Answer from the drawing. Dimensions are ordinates in mm from the lowest x, y and z of the part. Round coordinates to 2 decimals unless told otherwise and drop trailing zeros. Loops run counter-clockwise (first coordinate to the right, second up) from the corner with the lowest first, then second, coordinate; pieces in that order, holes last. Notation, with made-up numbers: (77.25, 1) - (121.25, 1) arc R27 ccw to (121.25, 17) - close; hole circle Ø11 at (-9, -6.75). An arc over 180 degrees is marked (long way). Return JSON: item names as keys, results as strings.
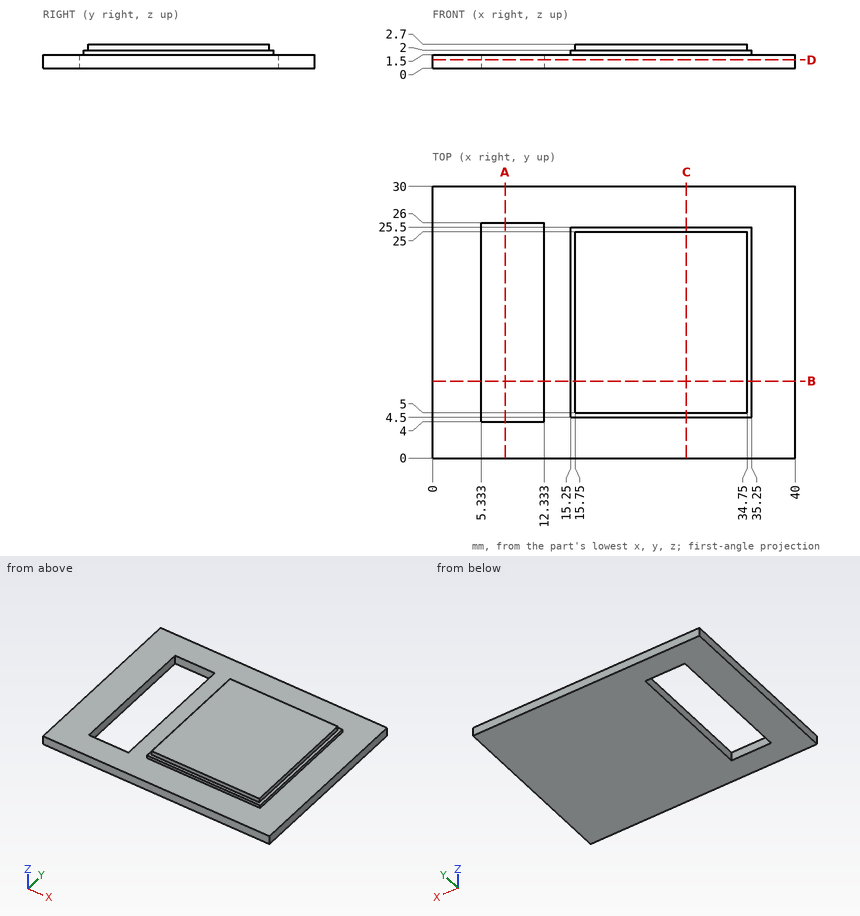
1) Flat-ended cylindrical pins translate along their axes: pin 1 (8 mm diameter, centred on x = 36, y = 14.5, fed in from +Z); pin 2 (8 mm diameter, centred on x = 6.5, y = 19, fed in from +Z); pin 3 (0.8 mm diameter, centred on x = 30, z = 2, fed in from -Y); pin 4 (0.6 mm diameter, centred on y = 11.5, z = 2, fed in from -X). Find the tip coordinate at first contact, or state that the pin passes through.
Verdict:
{"pin 1": "stops at z = 2.7", "pin 2": "stops at z = 1.5", "pin 3": "stops at y = 4.5", "pin 4": "stops at x = 15.25"}
2) Section C-C (x = 28) is taken. Give the vertices of the cut face in (y, z), and give its area (3 significant figures).
Verdict:
{"outline": "(0, 0) - (30, 0) - (30, 1.5) - (25.5, 1.5) - (25.5, 2) - (25, 2) - (25, 2.7) - (5, 2.7) - (5, 2) - (4.5, 2) - (4.5, 1.5) - (0, 1.5) - close", "area": "69.5 mm2"}
3) Find the intervals of material crossed by L1, parallel to Y at x = 6, z = 1.05; L2, parallel to X at y = 22.5, z = 1.3; L3, parallel to X at y = 19, z = 1.9, in increasing order.
Verdict:
{"L1": "y = 0 to 4, 26 to 30", "L2": "x = 0 to 5.33, 12.33 to 40", "L3": "x = 15.25 to 35.25"}
4) Section A-A (x = 8) is taken. Give the vertices of the cut face in (y, z), and give its area (3 significant figures).
Verdict:
{"outline": "(0, 0) - (4, 0) - (4, 1.5) - (0, 1.5) - close; (26, 0) - (30, 0) - (30, 1.5) - (26, 1.5) - close", "area": "12.0 mm2"}
5) Section D-D (z = 0.95) is taken. Give the vertices of the cut face in (x, y), and give its area (3 significant figures).
Verdict:
{"outline": "(0, 0) - (40, 0) - (40, 30) - (0, 30) - close; hole (5.33, 4) - (12.33, 4) - (12.33, 26) - (5.33, 26) - close", "area": "1,050 mm2"}
6) Section B-B (y = 8.5) is taken. Give the vertices of the cut face in (x, z).
Verdict:
{"outline": "(0, 0) - (5.33, 0) - (5.33, 1.5) - (0, 1.5) - close; (12.33, 0) - (40, 0) - (40, 1.5) - (35.25, 1.5) - (35.25, 2) - (34.75, 2) - (34.75, 2.7) - (15.75, 2.7) - (15.75, 2) - (15.25, 2) - (15.25, 1.5) - (12.33, 1.5) - close"}
